Source: three-view drawing plus pictorial views. Frame: mm from the lowest corner of the part. A direction names the side the tool comes from. Coordinates: 2 decimals unless noted, no trailing zeros. Order: outer loops, then holes, each group sorted by start corner. A loop starts at its lowest first (then second) coordinate and runs counter-clockwise, first axis right, second up. Notation, with made-up numbers: M -0.75,-14 L 51.25,-14 A19 ccw 51.25,-6 Z; hole C -2,6 d3. An arc over 180 degrees is marked long. One line per question, with ' | ' between items.
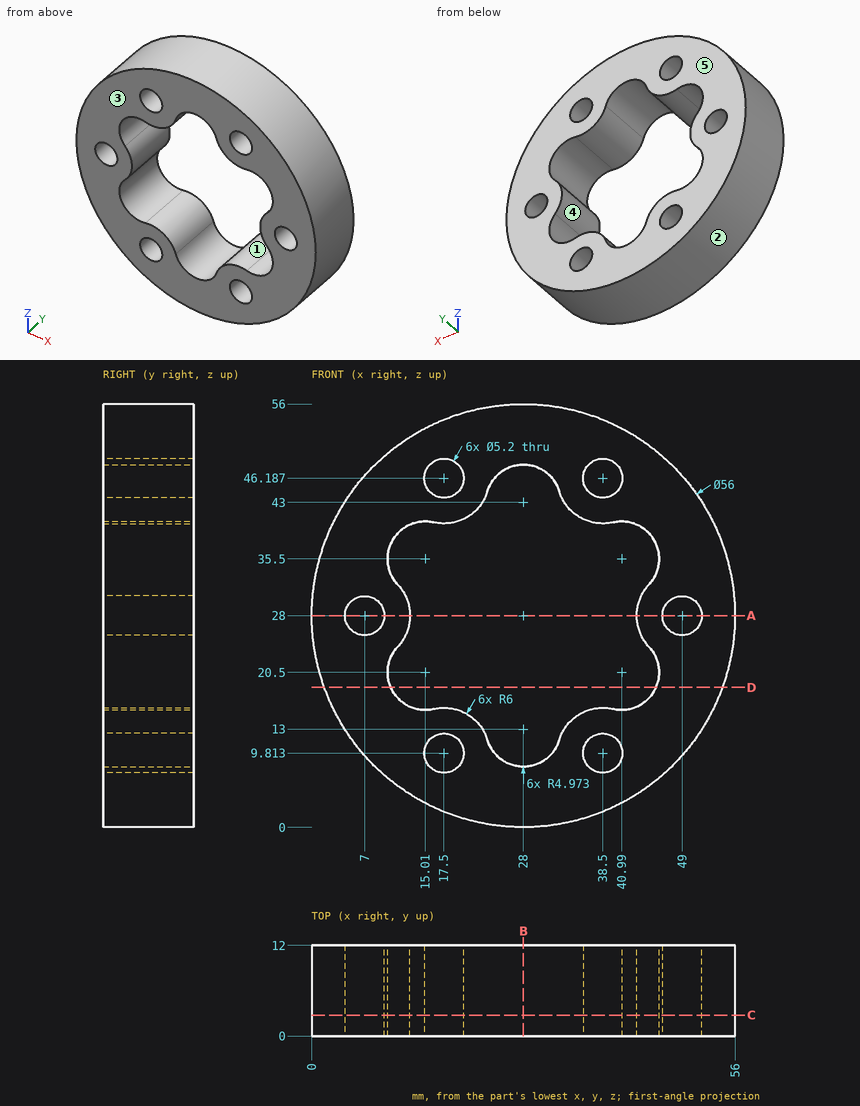
1. Access query for the marked faces 4 and 5. Directions: +Z, -Z, +X, -X, +Y, -Y. A direction counts if a zero-diameter tool reaches every point of the face in a straight line with its end or side. Return the directions, or none.
Response values:
face 4: +Y, -Y | face 5: +Z, -Z, +X, -X, +Y
2. Section B-B, the plane x = 28. Output: boundary loops of the cut face in (y, z).
Response values:
outline: M 0,0 L 12,0 L 12,8.03 L 0,8.03 Z; M 0,47.97 L 12,47.97 L 12,56 L 0,56 Z
3. Section D-D, the plane z = 18.5. Output: boundary loops of the cut face in (x, y).
Response values:
outline: M 1.66,0 L 10.46,0 L 10.46,12 L 1.66,12 Z; M 45.54,0 L 54.34,0 L 54.34,12 L 45.54,12 Z
4. Section A-A, the plane z = 28. Output: boundary loops of the cut face in (x, y), and give its area (3 significant figures).
Response values:
outline: M 0,0 L 4.4,0 L 4.4,12 L 0,12 Z; M 9.6,0 L 13,0 L 13,12 L 9.6,12 Z; M 43,0 L 46.4,0 L 46.4,12 L 43,12 Z; M 51.6,0 L 56,0 L 56,12 L 51.6,12 Z | area: 187 mm^2
5. Draft query along Z for the marked faces 1, 2 and 3. Return one class per face: pulls with the +Z half, pulls with the -Z half, needs draft (parallel to the pull), parting line crosses it, or undercut.
Response values:
face 1: undercut | face 2: parting line crosses it | face 3: needs draft
6. Section C-C, the plane y = 2.75. Output: boundary loops of the cut face in (x, z) (1 decimal), and give its area (3 significant figures).
Response values:
outline: C 28,28 d56; hole C 7,28 d5.2; hole M 11.4,23.9 A5 ccw 16.1,15.7 A6 cw 23.2,11.6 A5 ccw 32.8,11.6 A6 cw 39.9,15.7 A5 ccw 44.6,23.9 A6 cw 44.6,32.1 A5 ccw 39.9,40.3 A6 cw 32.8,44.4 A5 ccw 23.2,44.4 A6 cw 16.1,40.3 A5 ccw 11.4,32.1 A6 cw Z; hole C 17.5,9.8 d5.2; hole C 17.5,46.2 d5.2; hole C 38.5,9.8 d5.2; hole C 38.5,46.2 d5.2; hole C 49,28 d5.2 | area: 1,360 mm^2
7. Material intervals for line 1 (Z direction, x = 38.5, y = 5.75) (1 decimal); line 2 (Z direction, x = 19, y = 10.25) (1 decimal); line 3 (Z direction, x = 30, y = 4.5), sorted ascending. Write a range as [from, to].
Response values:
line 1: z = [2, 7.2], [12.4, 15.8], [40.2, 43.6], [48.8, 54] | line 2: z = [1.5, 7.7], [11.9, 15.6], [40.4, 44.1], [48.3, 54.5] | line 3: z = [0.07, 8.45], [47.55, 55.93]
8. Pin query (flat end, axial travel): P1, Ø1, axis at y = 6.5, z = 34.5, coming from the +X side; P2, Ø2, axis at y = 2.5, z = 9, coming from the +X side; P3, Ø3, axis at y = 7.5, z = 9.5, coming from the -X side. Return the tip coordinate at first contact, or that it passes through.
Response values:
P1: stops at x = 55.35 | P2: stops at x = 49.45 | P3: stops at x = 5.75
